Autodesk Inventor part; units mm, degrees
ref_plane "YZ Plane" through (0, 0, 0) normal (1, 0, 0) x (0, 1, 0)
ref_plane "XZ Plane" through (0, 0, 0) normal (0, 1, 0) x (-1, 0, 0)
ref_plane "XY Plane" through (0, 0, 0) normal (0, 0, 1) x (1, 0, 0)
sketch "Sketch1" plane through (0, 0, 0) normal (0, 0, 1) x (1, 0, 0)
  line L0 (-34.86, 0) -> (34.86, 0) construction
  line L1 (0, -34.86) -> (0, 34.86) construction
  line L2 (0, 0) -> (11.1575, 11.1575) construction
  line L3 (0, 0) -> (15.7791, 0) construction
  line L4 (0, 24.9) -> (16.8009, 24.9)
  line L5 (16.8009, 24.9) -> (16.8009, 21.2415)
  line L6 (16.8009, 21.2415) -> (19.0212, 19.0212)
  line L7 (24.9, 0) -> (24.9, 16.8009)
  line L8 (24.9, 16.8009) -> (21.2415, 16.8009)
  line L9 (21.2415, 16.8009) -> (19.0212, 19.0212)
  line L10 (0, -24.9) -> (16.8009, -24.9)
  line L11 (16.8009, -24.9) -> (16.8009, -21.2415)
  line L12 (16.8009, -21.2415) -> (19.0212, -19.0212)
  line L13 (24.9, 0) -> (24.9, -16.8009)
  line L14 (24.9, -16.8009) -> (21.2415, -16.8009)
  line L15 (21.2415, -16.8009) -> (19.0212, -19.0212)
  line L16 (0, 24.9) -> (-16.8009, 24.9)
  line L17 (-16.8009, 24.9) -> (-16.8009, 21.2415)
  line L18 (-16.8009, 21.2415) -> (-19.0212, 19.0212)
  line L19 (-24.9, 16.8009) -> (-21.2415, 16.8009)
  line L20 (-21.2415, 16.8009) -> (-19.0212, 19.0212)
  line L21 (0, -24.9) -> (-16.8009, -24.9)
  line L22 (-16.8009, -24.9) -> (-16.8009, -21.2415)
  line L23 (-16.8009, -21.2415) -> (-19.0212, -19.0212)
  line L24 (-21.2415, -16.8009) -> (-19.0212, -19.0212)
  line L25 (-24.9, -16.8009) -> (-21.2415, -16.8009)
  line L26 (-24.9, 0) -> (-24.9, -16.8009)
  line L27 (-24.9, 0) -> (-24.9, 16.8009)
  circle A0 centre (0, 0) radius 12.5
  dimension "d0" = 45
  dimension "d2" = 24.9
  dimension "d3" = 3.14
  dimension "d4" = 26.9
  dimension "d5" = 25
extrude "Extrusion1" add sketch "Sketch1" along normal blind 5
sketch "Sketch3" plane through (0, 0, 0) normal (0, 0, -1) x (-1, 0, 0)
  circle A0 centre (0, 0) radius 12.5
extrude "Extrusion3" add sketch "Sketch3" against normal blind 3
sketch "Sketch4" plane through (0, 0, 3) normal (0, 0, 1) x (1, 0, 0)
  circle A0 centre (0, 0) radius 12.5
  arc A1 (-2.4955, 9.5466) -> (0.05, 7.811) centre (0.05, 10.5454) ccw
  arc A2 (-2.4955, 9.5466) -> (-3.0679, 9.7469) centre (-2.8679, 9.4005) ccw
  line L0 (-3.0679, 9.7469) -> (-6.8321, 7.5736)
  arc A3 (-6.8321, 7.5736) -> (-6.9449, 6.9778) centre (-6.6321, 7.2272) ccw
  arc A4 (-6.7145, 3.9055) -> (-6.9449, 6.9778) centre (-9.0826, 5.2727) ccw
  arc A5 (2.5955, -9.5466) -> (0.05, -7.811) centre (0.05, -10.5454) ccw
  arc A6 (2.5955, -9.5466) -> (3.1679, -9.7469) centre (2.9679, -9.4005) ccw
  line L1 (3.1679, -9.7469) -> (6.9321, -7.5736)
  arc A7 (6.9321, -7.5736) -> (7.0449, -6.9778) centre (6.7321, -7.2272) ccw
  arc A8 (6.8145, -3.9055) -> (7.0449, -6.9778) centre (9.1826, -5.2727) ccw
  line L2 (5.3229, -1.93) -> (5.3229, -1.58)
  line L3 (5.3229, -1.58) -> (5.4719, -1.58)
  line L4 (6.0377, -2.56) -> (5.9268, -2.56)
  line L5 (5.9268, -2.56) -> (5.9268, -2.3679)
  line L6 (5.674, -1.93) -> (5.3229, -1.93)
  circle A9 centre (0.05, 0) radius 3.3699
  line L7 (1.2704, -6.4878) -> (4.6724, -4.4373)
  line L8 (4.6724, -4.4373) -> (5.9738, -6.5964)
  line L9 (5.9738, -6.5964) -> (2.5718, -8.647)
  line L10 (2.5718, -8.647) -> (1.2704, -6.4878)
  line L11 (-2.4718, 8.647) -> (-1.1704, 6.4878)
  line L12 (-1.1704, 6.4878) -> (-4.5724, 4.4373)
  line L13 (-4.5724, 4.4373) -> (-5.8738, 6.5964)
  line L14 (-5.8738, 6.5964) -> (-2.4718, 8.647)
  arc A10 (-3.5679, -10.6129) -> (-1.5646, -9.9119) centre (-2.8679, -9.4005) ccw
  line L15 (-3.5679, -10.6129) -> (-7.3321, -8.4396)
  arc A11 (-7.7266, -6.3542) -> (-7.3321, -8.4396) centre (-6.6321, -7.2272) ccw
  arc A12 (-7.7266, -6.3542) -> (-9.3412, -3.5577) centre (-9.0826, -5.2727) ccw
  arc A13 (-10.95, -2.1733) -> (-9.3412, -3.5577) centre (-9.55, -2.1733) ccw
  line L16 (-10.95, -2.1733) -> (-10.95, 2.1733)
  arc A14 (-9.3412, 3.5577) -> (-10.95, 2.1733) centre (-9.55, 2.1733) ccw
  arc A15 (-9.3412, 3.5577) -> (-7.7266, 6.3542) centre (-9.0826, 5.2727) ccw
  arc A16 (-7.3321, 8.4396) -> (-7.7266, 6.3542) centre (-6.6321, 7.2272) ccw
  line L17 (-7.3321, 8.4396) -> (-3.5679, 10.6129)
  arc A17 (-1.5646, 9.9119) -> (-3.5679, 10.6129) centre (-2.8679, 9.4005) ccw
  arc A18 (-1.5646, 9.9119) -> (1.6646, 9.9119) centre (0.05, 10.5454) ccw
  arc A19 (3.6679, 10.6129) -> (1.6646, 9.9119) centre (2.9679, 9.4005) ccw
  line L18 (3.6679, 10.6129) -> (7.4321, 8.4396)
  arc A20 (7.8266, 6.3542) -> (7.4321, 8.4396) centre (6.7321, 7.2272) ccw
  arc A21 (7.8266, 6.3542) -> (9.4412, 3.5577) centre (9.1826, 5.2727) ccw
  arc A22 (11.05, 2.1733) -> (9.4412, 3.5577) centre (9.65, 2.1733) ccw
  line L19 (11.05, 2.1733) -> (11.05, -2.1733)
  arc A23 (9.4412, -3.5577) -> (11.05, -2.1733) centre (9.65, -2.1733) ccw
  arc A24 (9.4412, -3.5577) -> (7.8266, -6.3542) centre (9.1826, -5.2727) ccw
  arc A25 (7.4321, -8.4396) -> (7.8266, -6.3542) centre (6.7321, -7.2272) ccw
  line L20 (7.4321, -8.4396) -> (3.6679, -10.6129)
  arc A26 (1.6646, -9.9119) -> (3.6679, -10.6129) centre (2.9679, -9.4005) ccw
  arc A27 (1.6646, -9.9119) -> (-1.5646, -9.9119) centre (0.05, -10.5454) ccw
  line L21 (-6.7145, 3.9055) -> (0.05, -7.811)
  line L22 (6.8145, -3.9055) -> (6.0377, -2.56)
  line L23 (5.9268, -2.3679) -> (5.674, -1.93)
  line L24 (5.4719, -1.58) -> (0.05, 7.811)
  dimension "d15" = 1
extrude "Extrusion4" add sketch "Sketch4" along normal up to surface (2 mm away) contours A0
properties part number "20_Cube_insert_Sample_holder"
For this review, take the finished solid that the model builds, in its own axes (mm). A direction names the side the tool comes from. Round coordinates to 2 decimals unless told otherwise and drop trailing zeros. Write each loop counter-clockwise with the first axis right and the second up, starting at its lowest first coordinate (ties: lowest second). Pieces come first, ordered by that corner, then holes. Notation, with made-up numbers: M 48.25,77.5 L 73.25,77.5 A17 cw 73.25,83.5 Z; hole C 36.25,15.5 d11. An arc over 180 degrees is marked long. Write item = value, one per line. Start each with the question number.
(1) We need section B-B (x = 0). Give the boundary of the cut face in (y, z).
(2) We need section A-A (z = 0.6). Give the boundary of the cut face in (x, y), then the cut area to 3 significant figures.
(3) Clearance check with flat-ended pins moving along their axes: pin 1 Ø1.1 at (y, z) = (23.5, 2) entering from -X; pin 2 Ø1.8 at (x, z) = (24, 2) entering from +Y; pin 3 Ø1.1 at (y, z) = (22.5, 3.5) entering from +X. State where each tip first meets the part, or that it passes through.
(4) We need section C-C (y = -22). Give the boundary of the cut face in (x, z).
(5) The part is to be moulded in two halves that separate along X. For faces 5 (the face through (-5.48, 9.51, 3.99)), 6 (the face through (16.801, -23, 2)), 7 (the face through (8.11, -7.47, 3.99)), 8 (the face through (-16.801, -23, 2)), say which applies: +X half, -X half, draft (parallel to the pull), parting line (faces both ways), or undercut.
(6) For faces 1 (the face through (23, 16.801, 2)), 2 (the face through (24.9, 0, 2)), 3 (the face through (5.524, 9.541, 3.986)), 4 (the face through (-16.801, 23, 2)), list the 3-axis set-ups (+Z, -Z, +X, -X, +Y, -Y) from which the entire face can be reached by the end or side of a thin tool; tool diameter is ignored.
(7) For line 1 along X through (y, z) = (-0.5, 3.3); line 2 along Y through (x, z) = (3, 4.75); line 3 along Y through (x, z) = (22, 4.65), list the stretches that pass through material, from the lowest coordinate up.
(8) We need section D-D (x = 18). Give the boundary of the cut face in (y, z).
Results found:
q1.outline = M -24.9,0 L 24.9,0 L 24.9,5 L 8.81,5 L 8.81,3 L -8.81,3 L -8.81,5 L -24.9,5 Z
q2.outline = M -24.9,-16.8 L -21.24,-16.8 L -16.8,-21.24 L -16.8,-24.9 L 16.8,-24.9 L 16.8,-21.24 L 21.24,-16.8 L 24.9,-16.8 L 24.9,16.8 L 21.24,16.8 L 16.8,21.24 L 16.8,24.9 L -16.8,24.9 L -16.8,21.24 L -21.24,16.8 L -24.9,16.8 Z
q2.area = 2,260 mm²
q3.pin_1 = -16.8
q3.pin_2 = 16.8
q3.pin_3 = 16.8
q4.outline = M -16.8,0 L 16.8,0 L 16.8,5 L -16.8,5 Z
q5.face_5 = undercut
q5.face_6 = +X half
q5.face_7 = undercut
q5.face_8 = -X half
q6.face_1 = +Z, -Z, +X, +Y
q6.face_2 = +Z, -Z, +X, +Y, -Y
q6.face_3 = +Z
q6.face_4 = +Z, -Z, -X, +Y
q7.line_1 = -24.9 to -10.95, 11.05 to 24.9
q7.line_2 = -24.9 to -10.8, 10.8 to 24.9
q7.line_3 = -16.8 to 16.8
q8.outline = M -20.04,0 L 20.04,0 L 20.04,5 L -20.04,5 Z
